Build history of the part. All positions in model axes, mm. A direction names the side the tool comes from. Coordinates: 2 decimals unless noted, no trailing zeros. Loops run counter-clockwise (first coordinate to the right, second up) from the corner with the lowest first, then second, coordinate; pieces in that order, holes last. Notation, with made-up numbers: (41, 25.5) -> (67, 25.5) arc R32 ccw to (67, 63.5) -> close; hole circle Ø2 at (-19.75, 77). An arc over 180 degrees is marked (long way). One line per item, written item: value. Start each with the question number.
```python
from build123d import *

# Parameters (mm, degrees)
SKETCH2_W               = 54
SKETCH2_H               = 200
SKETCH2_W_2             = 38
SKETCH2_H_2             = 184
BOSS_EXTRUDE2_DEPTH     = 55
CUT_EXTRUDE1_DEPTH      = 118.277448813
BOSS_EXTRUDE3_START     = 55
SKETCH5_W               = 54
SKETCH5_H               = 200
BOSS_EXTRUDE3_DEPTH     = 8
CUT_EXTRUDE2_DEPTH      = 122.235308388
CUT_EXTRUDE2_DEPTH_BACK = 122.235308388
SKETCH6_R               = 1.75
CUT_EXTRUDE3_START      = 63
SKETCH7_R               = 3
CUT_EXTRUDE3_DEPTH      = 44
CHAMFER1_SIZE           = 5
CHAMFER3_SIZE           = 5
CHAMFER4_SIZE           = 3
BOSS_EXTRUDE4_START     = -5
SKETCH8_R               = 1.75
BOSS_EXTRUDE4_DEPTH     = 5
CUT_EXTRUDE4_DEPTH      = 122.235308388
CUT_EXTRUDE4_DEPTH_BACK = 122.235308388
SKETCH9_W               = 6
SKETCH9_H               = 20
SKETCH10_W              = 10
SKETCH10_H              = 16
CUT_EXTRUDE5_DEPTH      = 122.235308388


with BuildPart() as part:
    # Sketch2 → Boss-Extrude2 (new body)
    with BuildSketch(Plane(origin=(0, 0, 0), x_dir=(1, 0, 0), z_dir=(0, 1, 0))):
        Rectangle(SKETCH2_W, SKETCH2_H)
        Rectangle(SKETCH2_W_2, SKETCH2_H_2, mode=Mode.SUBTRACT)
    extrude(amount=BOSS_EXTRUDE2_DEPTH)

    # Sketch3 → Cut-Extrude1 (cut, through all)
    with BuildSketch(Plane(origin=(0, 0, 0), x_dir=(0, 0, -1), z_dir=(1, 0, 0))):
        with BuildLine():
            Line((-51, 0), (-51, 31))
            ThreePointArc((-51, 31), (-40, 42), (-29, 31))
            Line((-29, 31), (-29, 0))
            Line((-29, 0), (-51, 0))
        make_face()
        with BuildLine():
            Line((51, 0), (51, 31))
            ThreePointArc((51, 31), (40, 42), (29, 31))
            Line((29, 31), (29, 0))
            Line((29, 0), (51, 0))
        make_face()
    extrude(amount=CUT_EXTRUDE1_DEPTH, mode=Mode.SUBTRACT)

    # Sketch5 → Boss-Extrude3 (add)
    with BuildSketch(Plane(origin=(0, 0, 0), x_dir=(1, 0, 0), z_dir=(0, 1, 0)).offset(BOSS_EXTRUDE3_START)):
        Rectangle(SKETCH5_W, SKETCH5_H)
    extrude(amount=BOSS_EXTRUDE3_DEPTH)

    # Sketch6 → Cut-Extrude2 (cut, two sides: drawn at the far end of the back side and taken through both)
    with BuildSketch(Plane(origin=(0, 0, 0), x_dir=(1, 0, 0), z_dir=(0, 1, 0)).offset(-CUT_EXTRUDE2_DEPTH_BACK)):
        with Locations(Location((22, -95, 0), (0, 0, 270))):
            Circle(SKETCH6_R)
        with Locations(Location((-22, -95, 0), (0, 0, 270))):
            Circle(SKETCH6_R)
        with Locations(Location((-22, 95, 0), (0, 0, 270))):
            Circle(SKETCH6_R)
        with Locations(Location((22, 95, 0), (0, 0, 270))):
            Circle(SKETCH6_R)
    extrude(amount=CUT_EXTRUDE2_DEPTH + CUT_EXTRUDE2_DEPTH_BACK, mode=Mode.SUBTRACT)

    # Sketch7 → Cut-Extrude3 (cut)
    with BuildSketch(Plane(origin=(0, 0, 0), x_dir=(1, 0, 0), z_dir=(0, 1, 0)).offset(CUT_EXTRUDE3_START)):
        with Locations(Location((-22, -95, 0), (0, 0, 90))):
            Circle(SKETCH7_R)
        with Locations(Location((-22, 95, 0), (0, 0, 90))):
            Circle(SKETCH7_R)
        with Locations(Location((22, 95, 0), (0, 0, 90))):
            Circle(SKETCH7_R)
        with Locations(Location((22, -95, 0), (0, 0, 90))):
            Circle(SKETCH7_R)
    extrude(amount=-CUT_EXTRUDE3_DEPTH, mode=Mode.SUBTRACT)

    # Chamfer1
    chamfer1_edges = [part.edges().sort_by_distance(p)[0] for p in [
        (-27, 31.5, -100),
        (27, 31.5, -100),
        (27, 31.5, 100),
        (-27, 31.5, 100),
    ]]
    chamfer(chamfer1_edges, length=CHAMFER1_SIZE)

    # Chamfer3
    # the kernel refuses this chamfer: 5 mm, written as the material it takes off along each edge
    with BuildSketch(Plane(origin=(-34.85841494, 63, 100), x_dir=(0, -0.9996219169112968, 0.0274958766105877), z_dir=(1, 0, 0))) as chamfer3_piece_1:
        Polygon((CHAMFER3_SIZE * 0.999621916911, CHAMFER3_SIZE * 0.0274958766106), (-CHAMFER3_SIZE * 0.0274958766106, CHAMFER3_SIZE * 0.999621916911), (0, 0), align=None)
    extrude(amount=69.71682988, mode=Mode.SUBTRACT)
    with BuildSketch(Plane(origin=(-27, 63, -107.85841494), x_dir=(0.9996219169112968, 0.027495876610586317, 0), z_dir=(0, 0, 1)), Plane(origin=(27, 63, 107.85841494), x_dir=(-0.9996219169112968, 0.027495876610586317, 0), z_dir=(0, 0, -1))) as chamfer3_piece_2:
        Polygon((CHAMFER3_SIZE * 0.999621916911, -CHAMFER3_SIZE * 0.0274958766106), (-CHAMFER3_SIZE * 0.0274958766106, -CHAMFER3_SIZE * 0.999621916911), (0, 0), align=None)
    extrude(amount=215.71682988, mode=Mode.SUBTRACT)
    with BuildSketch(Plane(origin=(34.85841494, 63, -100), x_dir=(0, 0.027495876610586282, 0.9996219169112968), z_dir=(-1, 0, 0))) as chamfer3_piece_3:
        Polygon((CHAMFER3_SIZE * 0.999621916911, -CHAMFER3_SIZE * 0.0274958766106), (-CHAMFER3_SIZE * 0.0274958766106, -CHAMFER3_SIZE * 0.999621916911), (0, 0), align=None)
    extrude(amount=69.71682988, mode=Mode.SUBTRACT)
    with BuildSketch(Plane(origin=(12.907727601, 63, 109.092272399), x_dir=(-0.7068394360706735, 0.027495876610586337, -0.7068394360706735), z_dir=(0.7071067811865476, 0, -0.7071067811865476)), Plane(origin=(36.092272399, 63, -85.907727601), x_dir=(-0.7068394360706735, 0.027495876610586334, 0.7068394360706735), z_dir=(-0.7071067811865476, 0, -0.7071067811865476))) as chamfer3_piece_4:
        Polygon((CHAMFER3_SIZE * 0.999621916911, -CHAMFER3_SIZE * 0.0274958766106), (-CHAMFER3_SIZE * 0.0274958766106, -CHAMFER3_SIZE * 0.999621916911), (0, 0), align=None)
    extrude(amount=32.787897692, mode=Mode.SUBTRACT)
    with BuildSketch(Plane(origin=(-36.092272399, 63, -85.907727601), x_dir=(0.7068394360706735, 0.027495876610586334, 0.7068394360706735), z_dir=(0.7071067811865476, 0, -0.7071067811865476)), Plane(origin=(-12.907727601, 63, 109.092272399), x_dir=(0.7068394360706735, 0.027495876610586337, -0.7068394360706735), z_dir=(-0.7071067811865476, 0, -0.7071067811865476))) as chamfer3_piece_5:
        Polygon((CHAMFER3_SIZE * 0.999621916911, CHAMFER3_SIZE * 0.0274958766106), (-CHAMFER3_SIZE * 0.0274958766106, CHAMFER3_SIZE * 0.999621916911), (0, 0), align=None)
    extrude(amount=32.787897692, mode=Mode.SUBTRACT)

    # Chamfer4
    chamfer4_edges = [part.edges().sort_by_distance(p)[0] for p in [
        (27, 15.5, 29),
        (27, 42, 40),
        (27, 15.5, 51),
        (27, 15.5, -51),
        (27, 42, -40),
        (27, 15.5, -29),
    ]]
    chamfer(chamfer4_edges, length=CHAMFER4_SIZE)

    # Sketch8 → Boss-Extrude4 (add)
    # profile 1 of 2: a face of its own
    with BuildSketch(Plane(origin=(0, 0, 0), x_dir=(1, 0, 0), z_dir=(0, 1, 0)).offset(BOSS_EXTRUDE4_START)):
        Polygon((27, -70), (19, -70), (19, -92), (-19, -92), (-19, -70), (-27, -70), (-27, -95), (-22, -100), (22, -100), (27, -95), align=None)
        with Locations(Location((22, -95, 0), (0, 0, 90))):
            Circle(SKETCH8_R, mode=Mode.SUBTRACT)
        with Locations(Location((-22, -95, 0), (0, 0, 90))):
            Circle(SKETCH8_R, mode=Mode.SUBTRACT)
    # profile 2 of 2: a face of its own
    with BuildSketch(Plane(origin=(0, 0, 0), x_dir=(1, 0, 0), z_dir=(0, 1, 0)).offset(BOSS_EXTRUDE4_START)):
        Polygon((27, 95), (27, 70), (19, 70), (19, 92), (-19, 92), (-19, 70), (-27, 70), (-27, 95), (-22, 100), (22, 100), align=None)
        with Locations(Location((-22, 95, 0), (0, 0, 90))):
            Circle(SKETCH8_R, mode=Mode.SUBTRACT)
        with Locations(Location((22, 95, 0), (0, 0, 90))):
            Circle(SKETCH8_R, mode=Mode.SUBTRACT)
    extrude(amount=BOSS_EXTRUDE4_DEPTH)

    # Sketch9 → Cut-Extrude4 (cut, two sides: drawn at the far end of the back side and taken through both)
    with BuildSketch(Plane.XY.offset(-CUT_EXTRUDE4_DEPTH_BACK)):
        with Locations((-9, 5)):
            Rectangle(SKETCH9_W, SKETCH9_H)
    extrude(amount=CUT_EXTRUDE4_DEPTH + CUT_EXTRUDE4_DEPTH_BACK, mode=Mode.SUBTRACT)

    # Sketch10 → Cut-Extrude5 (cut, through all)
    with BuildSketch(Plane(origin=(0, 0, 0), x_dir=(0, 0, -1), z_dir=(1, 0, 0))):
        with Locations((-75, 3)):
            Rectangle(SKETCH10_W, SKETCH10_H)
        with Locations((75, 3)):
            Rectangle(SKETCH10_W, SKETCH10_H)
    extrude(amount=CUT_EXTRUDE5_DEPTH, mode=Mode.SUBTRACT)


solid = part.part
```
Item 1: Tool access for faces 5 (the face through (21, 16, -29)), 6 (the face through (-20, 19, 95)), 7 (the face through (-23, -3, 70)), 8 (the face through (-6, 5, -96)): list every direction of +Z, -Z, +X, -X, +Y, -Y with a clear straight run to the whole face (end or side of a thin tool).
Item 2: Probe probe 1 along Z at (x, y) = (22, 50); probe 2 along X at (y, z) = (43.5, 95); probe 3 along Z at (x, y) = (-22, 10). List the from-to ranges inside material, lowest first.
Item 3: Band-saw the part on B-B, the plane x = 14. List the corners of the cut face in (y, z), and give its area (4 significant figures).
Item 4: Drop flat-ended pins along their axis: pin 1 Ø1.8 at (x, z) = (21.5, 94) entering from +Y; pin 2 Ø9 at (x, z) = (25, -75) entering from -Y; pin 3 Ø10 at (x, z) = (-19, 23) entering from -Y. Give the stop position or say it passes through.
Item 5: Two-plate mould, pull along X, no slides. Class faces 1 (the face through (23, 5, -70)), 2 (the face through (24, 26, 98)), 3 (the face through (-24.273, 58.37, -97.203)), 4 (the face through (-20.2, 41.3, -92.6)): +X half, -X half, draft (parallel to the pull), parting line (faces both ways), or undercut.
Item 6: Band-saw the part on A-A, the plane y = 9. Count the separate pieces of the cut face and the enclosed holes in it, and give its area (3 significant figures).
Item 7: Band-saw the part on C-C, the plane z = 9.5. List the corners of the cut face in (x, y), and give its area (3 significant figures).
Item 8: Band-saw the part on D-D, the plane z = 40. List the corners of the cut face in (x, y), and give its area (4 significant figures).
Worked out:
1. face 5: +X, -Y
1. face 6: +Y
1. face 7: +X, -X, -Y
1. face 8: +Z, -Z, -Y
2. probe 1: z = -100 to -98, -92 to 92, 98 to 100
2. probe 2: x = -27 to -25, -19 to 19, 25 to 27
2. probe 3: z = -100 to -96.75, -93.25 to 93.25, 96.75 to 100
3. outline: (-5, -100) -> (58, -100) -> (63, -95) -> (63, 95) -> (58, 100) -> (-5, 100) -> (-5, 92) -> (55, 92) -> (55, -92) -> (-5, -92) -> close
3. area: 2,535 mm²
4. pin 1: stops at y = 19
4. pin 2: stops at y = 11
4. pin 3: stops at y = 0
5. face 1: draft
5. face 2: +X half
5. face 3: -X half
5. face 4: undercut
6. separate pieces: 6
6. enclosed holes: 4
6. area: 3,090 mm²
7. outline: (-27, 0) -> (-19, 0) -> (-19, 55) -> (19, 55) -> (19, 0) -> (27, 0) -> (27, 58) -> (22, 63) -> (-22, 63) -> (-27, 58) -> close
7. area: 1,290 mm²
8. outline: (-27, 0) -> (-19, 0) -> (-19, 55) -> (19, 55) -> (19, 42) -> (24, 42) -> (27, 45) -> (27, 58) -> (22, 63) -> (-22, 63) -> (-27, 58) -> close
8. area: 946.5 mm²
